from build123d import *

# Parameters (mm, degrees)
BOSS_EXTRUDE1_START = -60.725
SKETCH1_W           = 32.8
SKETCH1_H           = 16.2
BOSS_EXTRUDE1_DEPTH = 10.275
BOSS_EXTRUDE2_START = -42.3
SKETCH2_W           = 42.2
SKETCH2_H           = 13
BOSS_EXTRUDE2_DEPTH = 2.3
BOSS_EXTRUDE3_START = 22.75
SKETCH3_R           = 6.5
BOSS_EXTRUDE3_DEPTH = 2.1
BOSS_EXTRUDE4_START = 22.75
SKETCH4_W           = 18.3
SKETCH4_H           = 13
BOSS_EXTRUDE4_DEPTH = 2.1
CUT_EXTRUDE1_START  = 22.75
SKETCH5_R           = 3.55
CUT_EXTRUDE1_DEPTH  = 2.1
CUT_EXTRUDE2_START  = 22.75
CUT_EXTRUDE2_DEPTH  = 2.1
BOSS_EXTRUDE5_START = -15.85
SKETCH7_R           = 6.5
BOSS_EXTRUDE5_DEPTH = 1.5
BOSS_EXTRUDE6_START = -15.85
SKETCH8_W           = 18.3
SKETCH8_H           = 13
BOSS_EXTRUDE6_DEPTH = 1.5
CUT_EXTRUDE3_START  = -15.85
SKETCH9_R           = 2.95
CUT_EXTRUDE3_DEPTH  = 1.5
CUT_EXTRUDE4_START  = -62.375
SKETCH10_W          = 23.2
SKETCH10_H          = 13
CUT_EXTRUDE4_DEPTH  = 8.625
CUT_EXTRUDE5_START  = -68
SKETCH11_R          = 1
CUT_EXTRUDE5_DEPTH  = 3
CUT_EXTRUDE6_START  = -68
SKETCH12_R          = 1
CUT_EXTRUDE6_DEPTH  = 3
CUT_EXTRUDE7_START  = -51.75
SKETCH13_R          = 3.15
CUT_EXTRUDE7_DEPTH  = 1.3
CUT_EXTRUDE8_START  = -10.7
SKETCH14_W          = 4.4
SKETCH14_H          = 6
CUT_EXTRUDE8_DEPTH  = 2.4


with BuildPart() as part:
    # Sketch1 → Boss-Extrude1 (new, symmetric)
    with BuildSketch(Plane(origin=(0, 0, 0), x_dir=(1, 0, 0), z_dir=(0, 1, 0)).offset(BOSS_EXTRUDE1_START)):
        with Locations((-24.7, 0)):
            Rectangle(SKETCH1_W, SKETCH1_H)
    extrude(amount=BOSS_EXTRUDE1_DEPTH, both=True)

    # Sketch2 → Boss-Extrude2 (add, symmetric)
    with BuildSketch(Plane(origin=(0, 0, 0), x_dir=(0, 0, -1), z_dir=(1, 0, 0)).offset(BOSS_EXTRUDE2_START)):
        with Locations((-3.75, -64.5)):
            Rectangle(SKETCH2_W, SKETCH2_H)
    extrude(amount=BOSS_EXTRUDE2_DEPTH, both=True)



with BuildPart() as body_2:
    # Sketch3 → Boss-Extrude3 (new, symmetric)
    with BuildSketch(Plane.XY.offset(BOSS_EXTRUDE3_START)):
        with Locations((-59.4, -64.5)):
            Circle(SKETCH3_R)
    extrude(amount=BOSS_EXTRUDE3_DEPTH, both=True)


with BuildPart() as part_1:
    add(part.part)

    add(body_2.part)  # Boss-Extrude4 merges body 2
    # Sketch4 → Boss-Extrude4 (add, symmetric)
    with BuildSketch(Plane.XY.offset(BOSS_EXTRUDE4_START)):
        with Locations((-50.25, -64.5)):
            Rectangle(SKETCH4_W, SKETCH4_H)
    extrude(amount=BOSS_EXTRUDE4_DEPTH, both=True)

    # Sketch5 → Cut-Extrude1 (cut, symmetric)
    with BuildSketch(Plane.XY.offset(CUT_EXTRUDE1_START)):
        with Locations((-59.4, -64.5)):
            Circle(SKETCH5_R)
    extrude(amount=CUT_EXTRUDE1_DEPTH, both=True, mode=Mode.SUBTRACT)

    # Sketch6 → Cut-Extrude2 (cut, symmetric)
    with BuildSketch(Plane.XY.offset(CUT_EXTRUDE2_START)):
        Polygon((-59.4, -60.95), (-46.7, -62.096718595), (-46.7, -66.903281405), (-59.4, -68.05), align=None)
    extrude(amount=CUT_EXTRUDE2_DEPTH, both=True, mode=Mode.SUBTRACT)



with BuildPart() as body_2_2:
    # Sketch7 → Boss-Extrude5 (new, symmetric)
    with BuildSketch(Plane.XY.offset(BOSS_EXTRUDE5_START)):
        with Locations((-59.4, -64.5)):
            Circle(SKETCH7_R)
    extrude(amount=BOSS_EXTRUDE5_DEPTH, both=True)


with BuildPart() as part_2:
    add(part_1.part)

    add(body_2_2.part)  # Boss-Extrude6 merges body 2 2
    # Sketch8 → Boss-Extrude6 (add, symmetric)
    with BuildSketch(Plane.XY.offset(BOSS_EXTRUDE6_START)):
        with Locations((-50.25, -64.5)):
            Rectangle(SKETCH8_W, SKETCH8_H)
    extrude(amount=BOSS_EXTRUDE6_DEPTH, both=True)

    # Sketch9 → Cut-Extrude3 (cut, symmetric)
    with BuildSketch(Plane.XY.offset(CUT_EXTRUDE3_START)):
        with Locations((-59.4, -64.5)):
            Circle(SKETCH9_R)
    extrude(amount=CUT_EXTRUDE3_DEPTH, both=True, mode=Mode.SUBTRACT)

    # Sketch10 → Cut-Extrude4 (cut, symmetric)
    with BuildSketch(Plane(origin=(0, 0, 0), x_dir=(1, 0, 0), z_dir=(0, 1, 0)).offset(CUT_EXTRUDE4_START)):
        with Locations((-24.7, 0)):
            Rectangle(SKETCH10_W, SKETCH10_H)
    extrude(amount=CUT_EXTRUDE4_DEPTH, both=True, mode=Mode.SUBTRACT)

    # Sketch11 → Cut-Extrude5 (cut, symmetric)
    with BuildSketch(Plane(origin=(0, 0, 0), x_dir=(1, 0, 0), z_dir=(0, 1, 0)).offset(CUT_EXTRUDE5_START)):
        with Locations(Location((-38.45, 0, 0), (0, 0, 270))):
            Circle(SKETCH11_R)
    extrude(amount=CUT_EXTRUDE5_DEPTH, both=True, mode=Mode.SUBTRACT)

    # Sketch12 → Cut-Extrude6 (cut, symmetric)
    with BuildSketch(Plane(origin=(0, 0, 0), x_dir=(1, 0, 0), z_dir=(0, 1, 0)).offset(CUT_EXTRUDE6_START)):
        with Locations(Location((-10.95, 0, 0), (0, 0, 270))):
            Circle(SKETCH12_R)
    extrude(amount=CUT_EXTRUDE6_DEPTH, both=True, mode=Mode.SUBTRACT)

    # Sketch13 → Cut-Extrude7 (cut, symmetric)
    with BuildSketch(Plane(origin=(0, 0, 0), x_dir=(1, 0, 0), z_dir=(0, 1, 0)).offset(CUT_EXTRUDE7_START)):
        with Locations(Location((-19.2, 0, 0), (0, 0, 270))):
            Circle(SKETCH13_R)
    extrude(amount=CUT_EXTRUDE7_DEPTH, both=True, mode=Mode.SUBTRACT)

    # Sketch14 → Cut-Extrude8 (cut, symmetric)
    with BuildSketch(Plane(origin=(0, 0, 0), x_dir=(0, 0, -1), z_dir=(1, 0, 0)).offset(CUT_EXTRUDE8_START)):
        with Locations((0, -56.75)):
            Rectangle(SKETCH14_W, SKETCH14_H)
    extrude(amount=CUT_EXTRUDE8_DEPTH, both=True, mode=Mode.SUBTRACT)


solid = part_2.part
For this review, take the finished solid that the model builds, in its own axes (mm). A direction names the side the tool comes from. Give positions to 0.01 mm unless a question says otherwise; leave off trailing zeros. Loops run counter-clockwise (first coordinate to the right, second up) from the corner with the lowest first, then second, coordinate; pieces in that order, holes last. Notation, with made-up numbers: M 28,86.5 L 33,86.5 A22 cw 33,112.5 Z; hole C 67,65.5 d7. An arc over 180 degrees is marked long. Answer as a JSON object with one key per item and string values. Group by question number.
Q1. Mouldability with a two-part tool opening along X and no side actions: class faces 5 (the cylindrical face through (-62.95, -64.41, 22.78)), 6 (the flat face through (-11, -59.75, 0)), 7 (the flat face through (-44.6, -64, 3)), 8 (the flat face through (-11, -65, 0)) as +X half, -X half, draft (parallel to the pull), parting line (faces both ways), or undercut.
Q2. Tool access review of faces 1 (the cylindrical face through (-21.995, -51.732, 1.454)), 2 (the flat face through (-40, -64, -13)), 3 (the flat face through (-41.1, -54, 0)), 4 (the flat face through (-46.7, -64, 23)): name each direction out of +Z, -Z, +X, -X, +Y, -Y from which nothing blocks a thin tool from reaching the whole face with its end or side.
Q3. Insertion check: P1, Ø10, axis at x = -37, y = -52.5, coming from the +Z side; P2, Ø10.5, axis at x = -31, y = -63, coming from the -Z side; P3, Ø6.5, axis at y = -64.5, z = 3, coming from the -X side. Each pin has a flat end and moves straight along its axis. Give the tip position at first contact, or say it passes through.
Q4. Add section D-D on x = -26.5. Give the boundary of the cut face in (y, z), and give its area (3 significant figures).
Q5. For probe 1 along Z at (x, y) = (-36, -54.75); probe 2 along Y at (x, z) = (-59.4, 22.65); probe 3 along Y at (x, z) = (-59.4, -15.75), list the stretches that pass through material, from the lowest coordinate up. Write a range as [from, to].
Q6. Add section B-B on x = -10.95. Give the boundary of the cut face in (y, z).
Q7. Add section C-C on y = -63.25. Give the boundary of the cut face in (x, z), and give its area (3 significant figures).
Q8. Add section A-A on z = 0. Give the boundary of the cut face in (x, y), and give its area (3 significant figures).
Checked values:
{
 "1": {"face 5": "undercut", "face 6": "draft", "face 7": "-X half", "face 8": "undercut"},
 "2": {"face 1": "+Y", "face 2": "-Z, +X, +Y, -Y", "face 3": "+Z, -Z, -X, +Y", "face 4": "+Z"},
 "3": {"P1": "z = 8.1", "P2": "z = -8.1", "P3": "x = -44.6"},
 "4": {"outline": "M -71,-8.1 L -50.45,-8.1 L -50.45,8.1 L -71,8.1 L -71,6.5 L -53.75,6.5 L -53.75,-6.5 L -71,-6.5 Z", "area": "109 mm²"},
 "5": {"probe 1": "[-8.1, -6.5], [6.5, 8.1]", "probe 2": "[-71, -68.05], [-60.95, -58]", "probe 3": "[-71, -67.45], [-61.55, -58]"},
 "6": {"outline": "M -71,-8.1 L -50.45,-8.1 L -50.45,8.1 L -71,8.1 L -71,1 L -65,1 L -65,-1 L -71,-1 Z; hole M -59.75,-2.2 L -53.75,-2.2 L -53.75,2.2 L -59.75,2.2 Z"},
 "7": {"outline": "M -65.78,-17.35 L -62.07,-17.35 L -62.07,-14.35 L -65.78,-14.35 Z; M -65.78,20.65 L -62.72,20.65 L -62.72,24.85 L -65.78,24.85 Z; M -56.73,-17.35 L -40,-17.35 L -40,-8.1 L -8.3,-8.1 L -8.3,8.1 L -40,8.1 L -40,24.85 L -46.7,24.85 L -46.7,20.65 L -44.6,20.65 L -44.6,-14.35 L -56.73,-14.35 Z; hole M -36.3,-6.5 L -13.1,-6.5 L -13.1,6.5 L -36.3,6.5 Z", "area": "475 mm²"},
 "8": {"outline": "M -44.6,-71 L -39.45,-71 L -39.45,-65 L -37.45,-65 L -37.45,-71 L -36.3,-71 L -36.3,-53.75 L -8.3,-53.75 L -8.3,-50.45 L -16.05,-50.45 L -16.05,-53.05 L -22.35,-53.05 L -22.35,-50.45 L -41.1,-50.45 L -41.1,-58 L -44.6,-58 Z; M -13.1,-71 L -11.95,-71 L -11.95,-65 L -9.95,-65 L -9.95,-71 L -8.3,-71 L -8.3,-59.75 L -13.1,-59.75 Z", "area": "250 mm²"}
}
